from build123d import *

# Parameters (mm, degrees)
SKETCH2_R           = 1
BOSS_EXTRUDE1_DEPTH = 1.6
FILLET1_R           = 3.8
SKETCH3_W           = 2.9
SKETCH3_H           = 10.72
CUT_EXTRUDE1_DEPTH  = 75.905340264
CUT_EXTRUDE2_DEPTH  = 75.905340264
FILLET2_R           = 0.5
LPATTERN1_COUNT     = 20
LPATTERN1_PITCH     = 2.75
CUT_EXTRUDE5_DEPTH  = 0.5
FILLET3_R           = 3
FILLET4_R           = 3.5
FILLET5_R           = 0.5
FILLET6_R           = 0.3


with BuildPart() as part:
    # Sketch2 → Boss-Extrude1 (new body)
    with BuildSketch(Plane(origin=(0, 0, 0), x_dir=(1, 0, 0), z_dir=(0, 1, 0))):
        with BuildLine():
            Line((0, 0), (0, 6))
            Line((0, 6), (4.5, 64))
            ThreePointArc((4.5, 64), (6.634239414, 69.95603241), (11.5, 74))
            Line((11.5, 74), (11.5, 13))
            Line((11.5, 13), (10, 0))
            Line((10, 0), (0, 0))
        make_face()
        with Locations(Location((6.6, 3.8, 0), (0, 0, 270))):
            Circle(SKETCH2_R, mode=Mode.SUBTRACT)
    extrude(amount=BOSS_EXTRUDE1_DEPTH)

    # Fillet1
    fillet1_edges = [part.edges().sort_by_distance(p)[0] for p in [
        (10, 0.8, 0),
    ]]
    fillet(fillet1_edges, radius=FILLET1_R)

    # Sketch3 → Cut-Extrude1 (cut, through all)
    with BuildSketch(Plane(origin=(0, 1.6, 0), x_dir=(1, 0, 0), z_dir=(0, 1, 0))):
        with Locations((1.45, 5.36)):
            Rectangle(SKETCH3_W, SKETCH3_H)
    extrude(amount=-CUT_EXTRUDE1_DEPTH, mode=Mode.SUBTRACT)

    # Sketch4 → Cut-Extrude2 (cut, through all)
    with BuildSketch(Plane(origin=(0, 1.6, 0), x_dir=(1, 0, 0), z_dir=(0, 1, 0))):
        Polygon((11.5, 69), (9.1, 68.125), (9.1, 67.125), (11.5, 66.25), align=None)
    cut_extrude2 = extrude(amount=-CUT_EXTRUDE2_DEPTH, mode=Mode.SUBTRACT)

    # Fillet2
    fillet2_edges = [part.edges().sort_by_distance(p)[0] for p in [
        (11.5, 0.8, -74),
    ]]
    fillet(fillet2_edges, radius=FILLET2_R)

    # LPattern1: Cut-Extrude2 ×20
    with Locations(*[(0, 0, i * LPATTERN1_PITCH) for i in range(1, LPATTERN1_COUNT)]):
        add(cut_extrude2, mode=Mode.SUBTRACT)

    # Sketch6 → Cut-Extrude5 (cut)
    with BuildSketch(Plane.XZ):
        with BuildLine():
            Line((5.74546219, -67.125), (4.930807018, -56.625))
            ThreePointArc((4.930807018, -56.625), (6.938890592, -61.750803415), (5.74546219, -67.125))
        make_face()
    extrude(amount=-CUT_EXTRUDE5_DEPTH, mode=Mode.SUBTRACT)

    # Fillet3
    # the kernel refuses this fillet: 3 mm, written as the material it adds along each edge
    with BuildSketch(Plane(origin=(-2.470700866, 0.5, -62.480857924), x_dir=(0.44582092023827286, 0, 0.8951221743862118), z_dir=(-0.8951221743862118, 0, 0.44582092023827286))) as fillet3_piece_1_section:
        with BuildLine():
            CenterArc((7.77955765, -3), FILLET3_R, 56.442690238, 33.557309762)
            Line((7.77955765, 0), (7.77955765, 0.06))
            Line((7.77955765, 0.06), (9.437870045, 0.06))
            Line((9.437870045, 0.06), (9.497870045, 0))
            ThreePointArc((9.497870045, 0), (9.497870045, -0.25), (9.471036293, -0.45))
            Line((9.471036293, -0.45), (9.437870045, -0.5))
        make_face()
    fillet3_piece_1 = revolve(axis=Axis((-2.470700866, 0.5, -62.480857924), (0, 1, 0)), revolution_arc=118.175305081, mode=Mode.PRIVATE)
    fillet3_piece_1 = split(fillet3_piece_1, bisect_by=Plane(origin=(5.338134618, 0.375117564, -61.875000174), z_dir=(0.997003710874575, 0, 0.07735373618854458)), keep=Keep.TOP, mode=Mode.PRIVATE)
    add(fillet3_piece_1)

    # Fillet4
    fillet4_edges = [part.edges().sort_by_distance(p)[0] for p in [
        (2.9, 0.8, 0),
    ]]
    fillet(fillet4_edges, radius=FILLET4_R)

    # Fillet5
    fillet5_edges = [part.edges().sort_by_distance(p)[0] for p in [
        (0.366206897, 0.8, -10.72),
    ]]
    fillet(fillet5_edges, radius=FILLET5_R)

    # Fillet6
    fillet6_edges = [part.edges().sort_by_distance(p)[0] for p in [
        (11.5, 0.8, -14),
        (2.9, 0.8, -10.72),
    ]]
    fillet(fillet6_edges, radius=FILLET6_R)


solid = part.part
Can you work these out from the model? Positions are in its coordinate system, mm. A direction names the side the tool comes from. Round coordinates to 2 decimals unless told otherwise and drop trailing zeros. Write each loop counter-clockwise with the first axis right and the second up, starting at its lowest first coordinate (ties: lowest second). Pieces come first, ordered by that corner, then holes. Notation, with made-up numbers: M -33.5,-13 L 24.5,-13 A23 ccw 24.5,22 Z; hole C -39.5,-19.5 d9. An arc over 180 degrees is marked long. Use a Markdown table: item, result.
Item 1: Which directions (+Z, -Z, +X, -X, +Y, -Y) give clear straight access to the entire face, cutting with the end or side of a thin tool? Please do faces 4 (the face through (2.9, 1, -7)), 5 (the face through (10.283, 0.811, -41.944)).
Found:
| item | result |
|---|---|
| face 4 | +Z, -X, +Y, -Y |
| face 5 | +X, +Y, -Y |
Item 2: For pin 1 Ø0.5 at (y, z) = (0.5, -37.5) entering from +X; pin 2 Ø0.5 at (x, y) = (2, 1) entering from +Z, each with a flat end and sliding along its axis, tell me the tip position at first contact or that it passes through.
Found:
| item | result |
|---|---|
| pin 1 | stops at x = 9.1 |
| pin 2 | stops at z = -10.72 |
Item 3: We'd pull the mould along Z, two halves only. Please class faces 1 (the face through (10.283, 0.811, -66.694)), 2 (the face through (6, 0, -29)), 3 (the face through (6.358, 0.789, -69.544)): released by +Z, released by -Z, zero draft, split by the parting line, or undercut.
Found:
| item | result |
|---|---|
| face 1 | undercut |
| face 2 | zero draft |
| face 3 | released by -Z |
Item 4: I want a section at A-A (x = 3.75). List the corners of the cut face in (y, z) for me, and give its area (3 significant figures).
Found:
| item | result |
|---|---|
| outline | M 0,-54.33 L 1.6,-54.33 L 1.6,-1.21 L 0,-1.21 Z |
| area | 85.0 mm2 |
Item 5: If I drill on line 1 along X through (y, z) = (0.55, -3.8); line 2 along Z through (x, y) = (6.5, 0.9); line 3 along X through (y, z) = (0.25, -35), over which ranges is the centre line in solid material (lowest first)? Write a range as [from, to].
Found:
| item | result |
|---|---|
| line 1 | x = [2.9, 5.6], [7.6, 10.44] |
| line 2 | z = [-69.76, -4.79], [-2.81, 0] |
| line 3 | x = [2.25, 9.1] |
